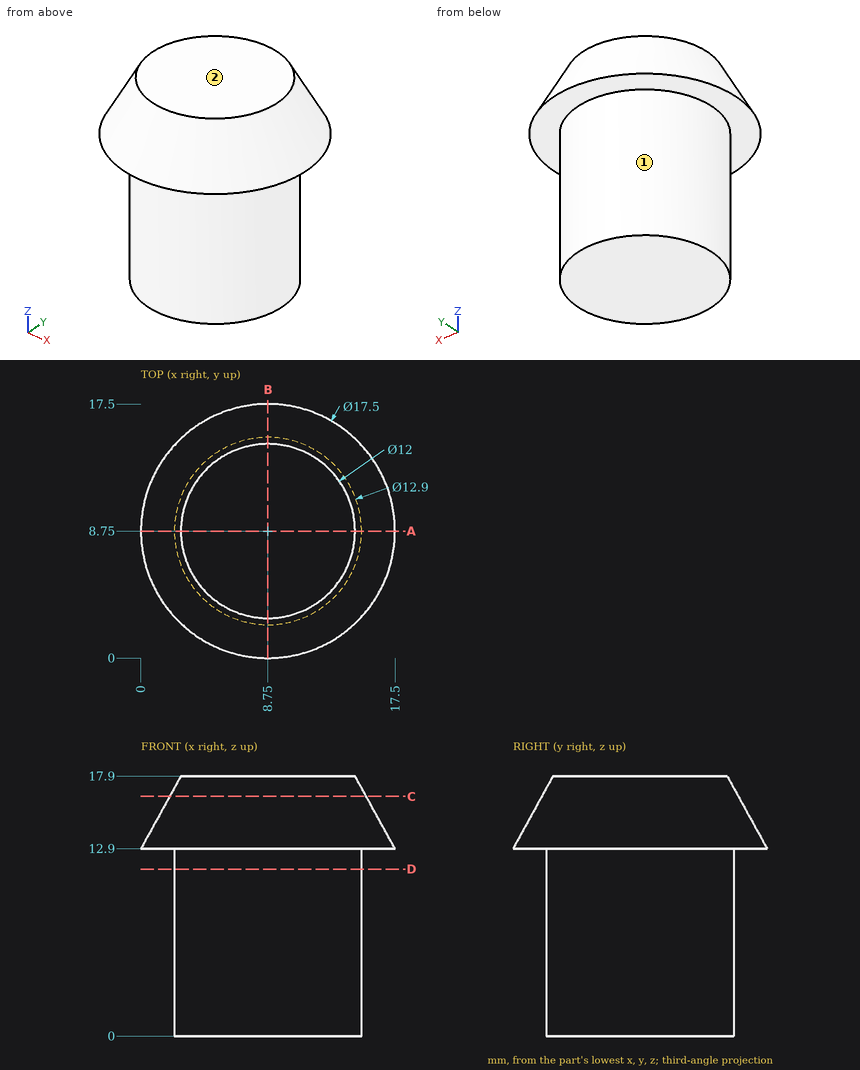
Source: three-view drawing plus pictorial views. Frame: mm from the lowest corner of the part. A direction names the side the tool comes from. Give positions to 0.01 mm unless a question says otherwise; leave off trailing zeros. Loops run counter-clockwise (first coordinate to the right, second up) from the corner with the lowest first, then second, coordinate; pieces in that order, holes last. Notation, with made-up numbers: (-11.5, 65) -> (30.5, 65) arc R19 cw to (30.5, 78) -> close; hole circle Ø4 at (-22, 12). An arc over 180 degrees is marked (long way). Use a Markdown table: item, result. Add a question column.
(1) Section query C-C (z = 16.5). Output: boundary loops of the cut face in (x, y), then the cut area to 3 significant figures.
(2) Section query D-D (z = 11.5). Output: boundary loops of the cut face in (x, y).
(3) Access query for the marked faces 1 and 2. Directions: +Z, -Z, +X, -X, +Y, -Y. A direction counts if a zero-diameter tool reaches every point of the face in a straight line with its end or side. Return the directions, or none.
(4) First-contact query: pin 1 Ø1 at (x, z) = (11.5, 15) entering from -Y; pin 2 Ø5 at (y, z) = (15, 12.5) entering from -X; pin 3 Ø1.5 at (x, z) = (10.5, 7.5) entering from +Y. Flat tips, straight axial feed; report the tip coordinate or a pass-through.
(5) Ray query, line 1 (Y direction, x = 8.75, z = 12); line 2 (Y direction, x = 3, z = 12.25). Return the intervals inside material, ascending.
(6) Section query A-A (y = 8.75). Output: boundary loops of the cut face in (x, z), then the cut area to 3 significant figures.
Checked values:
| question | item | result |
|---|---|---|
| 1 | outline | circle Ø13.54 at (8.75, 8.75) |
| 1 | area | 144 mm^2 |
| 2 | outline | circle Ø12.9 at (8.75, 8.75) |
| 3 | face 1 | -Z |
| 3 | face 2 | +Z, +X, -X, +Y, -Y |
| 4 | pin 1 | y = 1.33 |
| 4 | pin 2 | x = 0.86 |
| 4 | pin 3 | y = 15.12 |
| 5 | line 1 | 2.3 to 15.2 |
| 5 | line 2 | 5.83 to 11.67 |
| 6 | outline | (0, 12.9) -> (2.3, 12.9) -> (2.3, 0) -> (15.2, 0) -> (15.2, 12.9) -> (17.5, 12.9) -> (14.75, 17.9) -> (2.75, 17.9) -> close |
| 6 | area | 240 mm^2 |
